from build123d import *

# Parameters (mm, degrees)
SKETCH_1_R          = 35.5
SKETCH_1_R_2        = 2.6
EXTRUDE_2_DEPTH     = 1.9
EXTRUDE_START       = 4
SKETCH_3_R          = 37.5
SKETCH_3_R_2        = 2.6
EXTRUDE_3_DEPTH     = 4
SKETCH_2_W          = 13
SKETCH_2_H          = 6
CUT_EXTRUDE_6_DEPTH = 4
SKETCH_4_R          = 44.5
SKETCH_4_R_2        = 2
EXTRUDE_4_DEPTH     = 10
SKETCH_7_R          = 2.6
CUT_EXTRUDE_7_DEPTH = 65.910014636
SKETCH_10_R         = 5
CUT_EXTRUDE_8_DEPTH = 6.18
SKETCH_12_R         = 2
EXTRUDE_6_DEPTH     = 2
CUT_EXTRUDE_9_DEPTH = 2.5


with BuildPart() as part:
    # 草图1 → 凸台-拉伸2 (new body)
    with BuildSketch(Plane.XY):
        with Locations(Location((0, 0, 0), (0, 0, 180))):
            Circle(SKETCH_1_R)
        with Locations(Location((-27, 16, 0), (0, 0, 180))):
            Circle(SKETCH_1_R_2, mode=Mode.SUBTRACT)
        with Locations(Location((-27, -16, 0), (0, 0, 180))):
            Circle(SKETCH_1_R_2, mode=Mode.SUBTRACT)
        with Locations(Location((27, -16, 0), (0, 0, 180))):
            Circle(SKETCH_1_R_2, mode=Mode.SUBTRACT)
        with Locations(Location((27, 16, 0), (0, 0, 180))):
            Circle(SKETCH_1_R_2, mode=Mode.SUBTRACT)
    extrude(amount=EXTRUDE_2_DEPTH)

    # 草图3 → 凸台-拉伸3 (add)
    with BuildSketch(Plane(origin=(0, 0, 0), x_dir=(-1, 0, 0), z_dir=(0, 0, -1)).offset(EXTRUDE_START)):
        Circle(SKETCH_3_R)
        with Locations((27, 16)):
            Circle(SKETCH_3_R_2, mode=Mode.SUBTRACT)
        with Locations((27, -16)):
            Circle(SKETCH_3_R_2, mode=Mode.SUBTRACT)
        with Locations((-27, -16)):
            Circle(SKETCH_3_R_2, mode=Mode.SUBTRACT)
        with Locations((-27, 16)):
            Circle(SKETCH_3_R_2, mode=Mode.SUBTRACT)
    extrude(amount=-EXTRUDE_3_DEPTH)

    # 草图2 → 切除-拉伸6 (cut)
    with BuildSketch(Plane.XY.offset(1.9)):
        with Locations((12.7, 0)):
            Rectangle(SKETCH_2_W, SKETCH_2_H)
    extrude(amount=-CUT_EXTRUDE_6_DEPTH, mode=Mode.SUBTRACT)

    # 草图4 → 凸台-拉伸4 (add)
    with BuildSketch(Plane(origin=(0, 0, -4), x_dir=(-1, 0, 0), z_dir=(0, 0, -1))):
        Circle(SKETCH_4_R)
        with Locations((0, 40.5)):
            Circle(SKETCH_4_R_2, mode=Mode.SUBTRACT)
        with Locations((35.074028853, 20.25)):
            Circle(SKETCH_4_R_2, mode=Mode.SUBTRACT)
        with Locations((35.074028853, -20.25)):
            Circle(SKETCH_4_R_2, mode=Mode.SUBTRACT)
        with Locations((0, -40.5)):
            Circle(SKETCH_4_R_2, mode=Mode.SUBTRACT)
        with Locations((-35.074028853, -20.25)):
            Circle(SKETCH_4_R_2, mode=Mode.SUBTRACT)
        with Locations((-35.074028853, 20.25)):
            Circle(SKETCH_4_R_2, mode=Mode.SUBTRACT)
    extrude(amount=EXTRUDE_4_DEPTH)

    # 草图7 → 切除-拉伸7 (cut, through all)
    with BuildSketch(Plane.XY.offset(1.9)):
        with Locations(Location((27, -16, 0), (0, 0, 180))):
            Circle(SKETCH_7_R)
        with Locations(Location((27, 16, 0), (0, 0, 180))):
            Circle(SKETCH_7_R)
        with Locations(Location((-27, -16, 0), (0, 0, 180))):
            Circle(SKETCH_7_R)
        with Locations(Location((-27, 16, 0), (0, 0, 180))):
            Circle(SKETCH_7_R)
    extrude(amount=-CUT_EXTRUDE_7_DEPTH, mode=Mode.SUBTRACT)

    # 草图10 → 切除-拉伸8 (cut)
    with BuildSketch(Plane(origin=(0, 0, -14), x_dir=(-1, 0, 0), z_dir=(0, 0, -1))):
        with Locations((-27, 16)):
            Circle(SKETCH_10_R)
        with Locations(Location((27, 16, 0), (0, 0, 180))):
            Circle(SKETCH_10_R)
        with Locations((27, -16)):
            Circle(SKETCH_10_R)
        with Locations(Location((-27, -16, 0), (0, 0, 180))):
            Circle(SKETCH_10_R)
    extrude(amount=-CUT_EXTRUDE_8_DEPTH, mode=Mode.SUBTRACT)

    # 草图12 → 凸台-拉伸6 (add)
    with BuildSketch(Plane.XY.offset(-4)):
        with Locations((35.074028853, -20.25)):
            Circle(SKETCH_12_R)
        with Locations((35.074028853, 20.25)):
            Circle(SKETCH_12_R)
        with Locations((0, 40.5)):
            Circle(SKETCH_12_R)
        with Locations((-35.074028853, 20.25)):
            Circle(SKETCH_12_R)
        with Locations((-35.074028853, -20.25)):
            Circle(SKETCH_12_R)
        with Locations((0, -40.5)):
            Circle(SKETCH_12_R)
    extrude(amount=-EXTRUDE_6_DEPTH)

    # 草图13 → 切除-拉伸9 (cut)
    with BuildSketch(Plane(origin=(0, 0, -14), x_dir=(-1, 0, 0), z_dir=(0, 0, -1))):
        Polygon((47.534196194, -12), (42.851487722, -12), (36.070038026, -12), (31.570038026, -12), (31.570038026, -10), (28.361849592, -10), (28.361849592, 10), (31.570038026, 10), (31.570038026, 12), (36.070038026, 12), (42.851487722, 12), (47.534196194, 12), align=None)
    extrude(amount=-CUT_EXTRUDE_9_DEPTH, mode=Mode.SUBTRACT)


solid = part.part
Build history of the part. All positions in model axes, mm. A direction names the side the tool comes from. Coordinates: 2 decimals unless noted, no trailing zeros. Order: outer loops, then holes, each group sorted by start corner. A loop starts at its lowest first (then second) coordinate and runs counter-clockwise, first axis right, second up. Notation, with made-up numbers: (19, 11.25) - (72, 11.25) arc R26 ccw to (72, 39.25) - close; hole circle Ø9 at (-28.75, -31). An arc over 180 degrees is marked (long way). Write each question's results on one line, items separated by ' | '. Start each with the question number.
Item 1: Band-saw the part on C-C on x = 0. Write the cut outline in (y, z).
Item 2: Tool access for faces 1 (the face through (13, 3, 0)), 2 (the face through (36.55, -18.9, -9.94)), 3 (the face through (-30, 10, -13)): list every direction of +Z, -Z, +X, -X, +Y, -Y with a clear straight run to the whole face (end or side of a thin tool).
Item 3: Band-saw the part on A-A on x = 27. Write the cut outline in (y, z), and give its area (3 significant figures).
Item 4: Flat gauge pins, fed straight in: pin 1 (2 mm diameter, centred on x = 0.5, y = 41.5, fed in from -Z); pin 2 (6 mm diameter, centred on x = 3, z = -3.5, fed in from -Y); pin 3 (1.2 mm diameter, centred on x = -0.5, y = -39.5, fed in from -Z); pin 4 (1.5 mm diameter, centred on x = -34, z = -8, fed in from +Y). Where does each tip first touch, or does it go through?
Item 5: Mould opens along X. For faces 4 (the face through (36.55, 21.6, -9.94)), 5 (the face through (-37, 0, -11.5)), 6 (the face through (4.88, 37.18, -2.03)) say: released by +X, released by -X, zero draft, split by the parting line, or undercut.
Item 6: Wall check: probe 1 along Y at (x, z) = (0, -10.5); probe 2 along Y at (x, z) = (-27, -11.5); probe 3 along X at (y, z) = (-16, -0.5). Give the ranges that are in metal, low to high. Write a range as [from, to].
Item 7: Band-saw the part on B-B on y = 16. Write the cut outline in (x, z), and give its area (3 significant figures).
Item 8: Band-saw the part on D-D on y = -25.5. Write the cut outline in (x, z).
Numbers:
1) outline: (-44.5, -14) - (-42.5, -14) - (-42.5, -6) - (-38.5, -6) - (-38.5, -14) - (38.5, -14) - (38.5, -6) - (42.5, -6) - (42.5, -14) - (44.5, -14) - (44.5, -4) - (37.5, -4) - (37.5, 0) - (35.5, 0) - (35.5, 1.9) - (-35.5, 1.9) - (-35.5, 0) - (-37.5, 0) - (-37.5, -4) - (-44.5, -4) - close
2) face 1: +Z | face 2: -Z | face 3: -Z, -X
3) outline: (-35.37, -14) - (-21, -14) - (-21, -7.82) - (-18.6, -7.82) - (-18.6, 1.9) - (-23.05, 1.9) - (-23.05, 0) - (-26.02, 0) - (-26.02, -4) - (-35.37, -4) - close; (-13.4, -7.82) - (-11, -7.82) - (-11, -14) - (11, -14) - (11, -7.82) - (13.4, -7.82) - (13.4, 1.9) - (-13.4, 1.9) - close; (18.6, -7.82) - (21, -7.82) - (21, -14) - (35.37, -14) - (35.37, -4) - (26.02, -4) - (26.02, 0) - (23.05, 0) - (23.05, 1.9) - (18.6, 1.9) - close | area: 779 mm^2
4) pin 1: z = -14 | pin 2: y = -44.5 | pin 3: z = -6 | pin 4: y = 29.58
5) face 4: undercut | face 5: zero draft | face 6: split by the parting line
6) probe 1: [-44.5, -42.5], [-38.5, 38.5], [42.5, 44.5] | probe 2: [-35.37, -21], [-11, 11], [21, 35.37] | probe 3: [-33.92, -29.6], [-24.4, 24.4], [29.6, 33.92]
7) outline: (-41.52, -14) - (-32, -14) - (-32, -7.82) - (-29.6, -7.82) - (-29.6, 1.9) - (-31.69, 1.9) - (-31.69, 0) - (-33.92, 0) - (-33.92, -4) - (-41.52, -4) - close; (-24.4, -7.82) - (-22, -7.82) - (-22, -14) - (22, -14) - (22, -7.82) - (24.4, -7.82) - (24.4, 1.9) - (-24.4, 1.9) - close; (29.6, -7.82) - (32, -7.82) - (32, -14) - (41.52, -14) - (41.52, -4) - (33.92, -4) - (33.92, 0) - (31.69, 0) - (31.69, 1.9) - (29.6, 1.9) - close | area: 998 mm^2
8) outline: (-36.47, -14) - (36.47, -14) - (36.47, -4) - (27.5, -4) - (27.5, 0) - (24.7, 0) - (24.7, 1.9) - (-24.7, 1.9) - (-24.7, 0) - (-27.5, 0) - (-27.5, -4) - (-36.47, -4) - close
